Study the drawing (mm; zero at the part's minimum x, y, z) and answer. Coordinates: 2 decimals unless noted, no trailing zeros. Loops run counter-clockwise (first coordinate to the right, second up) from the corner with the lowest first, then second, coordinate; pieces in that order, holes last. Notation, with made-up numbers: (-18, -12) - (3, -12) arc R31 ccw to (3, 12) - close; hole circle Ø3 at (18, 69). An arc over 180 degrees is marked (long way). Use one line per item in the form item = value. Start each with the question number.
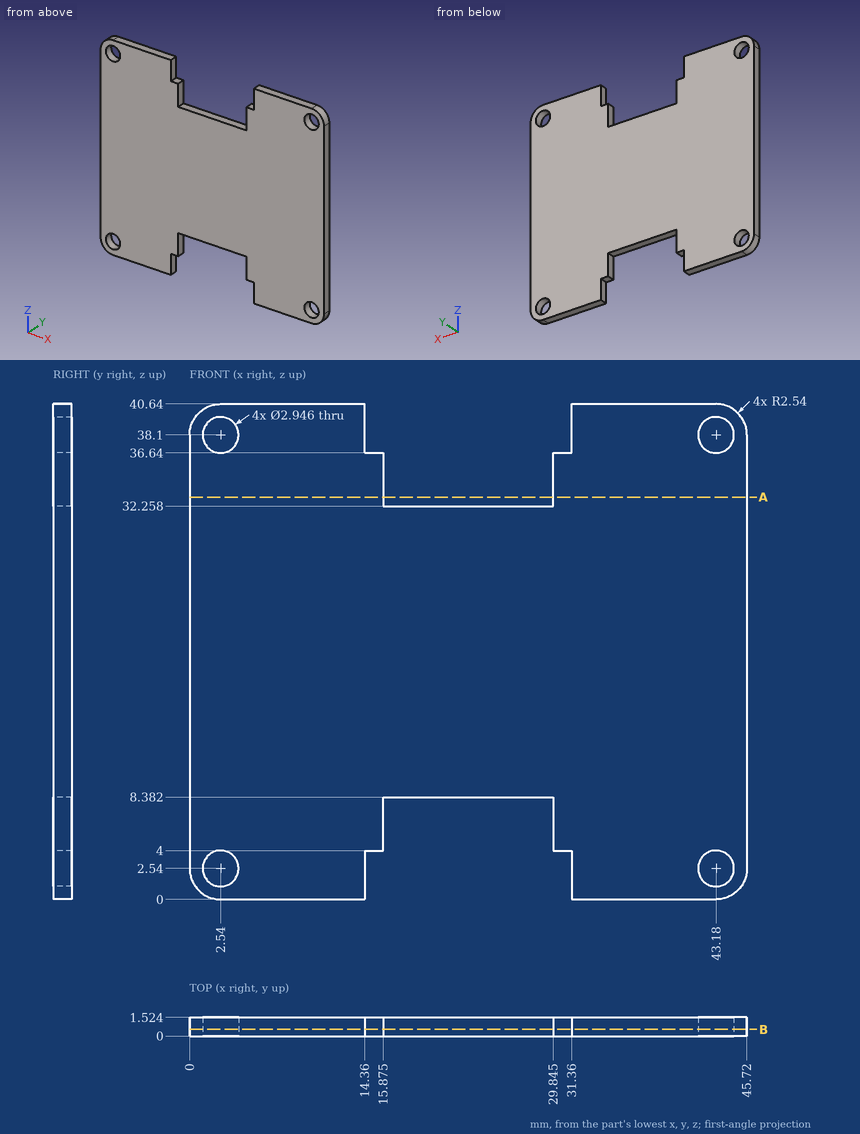
(1) A cutting plane is placed at A-A (z = 33). Determine the outline of the cut face in (x, y) (1 decimal).
(2) A cutting plane is placed at B-B (y = 0.55). Determine the outline of the cut face in (x, z) (1 decimal).
(3) Each of these flat-tipped pins is pushed along its axis until it touches: pin 1 Ø1.8 at (x, z) = (43.18, 2.54) entering from +Y; pin 2 Ø0.5 at (x, y) = (24, 1) entering from +Z; pin 3 Ø0.8 at (x, y) = (26, 1) entering from -Z; pin 4 Ø0.8 at (x, y) = (30.5, 0.5) entering from +Z. Where does it stop, or does it pass through?
(4) Find the intervals of material crossed by probe 1 along Z at (x, y) = (2.54, 1.05); probe 2 along X at (y, z) = (1.05, 2.54), in increasing order. Write a range as from..to.
Evaluation:
q1.outline = (0, 0) - (15.9, 0) - (15.9, 1.5) - (0, 1.5) - close; (29.8, 0) - (45.7, 0) - (45.7, 1.5) - (29.8, 1.5) - close
q2.outline = (0, 2.5) arc R2.5 ccw to (2.5, 0) - (14.4, 0) - (14.4, 4) - (15.9, 4) - (15.9, 8.4) - (29.8, 8.4) - (29.8, 4) - (31.4, 4) - (31.4, 0) - (43.2, 0) arc R2.5 ccw to (45.7, 2.5) - (45.7, 38.1) arc R2.5 ccw to (43.2, 40.6) - (31.4, 40.6) - (31.4, 36.6) - (29.8, 36.6) - (29.8, 32.3) - (15.9, 32.3) - (15.9, 36.6) - (14.4, 36.6) - (14.4, 40.6) - (2.5, 40.6) arc R2.5 ccw to (0, 38.1) - close; hole circle Ø2.9 at (2.5, 2.5); hole circle Ø2.9 at (2.5, 38.1); hole circle Ø2.9 at (43.2, 2.5); hole circle Ø2.9 at (43.2, 38.1)
q3.pin_1 = through
q3.pin_2 = 32.26
q3.pin_3 = 8.38
q3.pin_4 = 36.64
q4.probe_1 = 0..1.07, 4.01..36.63, 39.57..40.64
q4.probe_2 = 0..1.07, 4.01..14.36, 31.36..41.71, 44.65..45.72
